Check sheet for the modelled part. Datum: model origin and axes. Units: mm. Face numbers are marked on the shaded views. A direction names the side the tool comes from. Round coordinates to 2 decimals unless told otherwise and drop trailing zeros. Order: outer loops, then holes, each group sorted by start corner. A loop starts at its lowest first (then second) coordinate and runs counter-clockwise, first axis right, second up.
(1) Sectioned sample at C-C, the plane x = 4.5. Enter the section's corners in (y, z).
(2) Thickness scan on probe 1 along Y at (x, z) = (19.5, 10); probe 2 along X at (y, z) = (-5, 19); probe 3 along Y at (x, z) = (-28.5, 9). Record the ranges inside material, lowest first.
(3) Sectioned sample at A-A, the plane y = 4. Enter the section's corners in (x, z), and give its area (3 significant figures).
(4) Sectioned sample at B-B, the plane z = 15.5. Enter the section's corners in (x, y).
(5) Depth check by flat-ended pin: pin 1 (1.5 mm diameter, centred on x = 1.5, y = 6, fed in from +Z); pin 2 (1 mm diameter, centred on x = 0.5, y = 0, fed in from -Z); pin 3 (10 mm diameter, centred on x = 8.5, y = -2.5, fed in from +Z). Enter the tip coordinate at first touch or a pass-through.
(6) Mould release check, pull along X, two halves, no side actions. Record for the marked faces 1, 2 and 3: released by +X, released by -X, zero draft, split by the parting line, or undercut.
(7) Tool access check on the marked faces 4 and 5. Record the directions out of +Z, -Z, +X, -X, +Y, -Y that give a thin tool (end or side, any length) a straight path to the whole face; none if there is none.
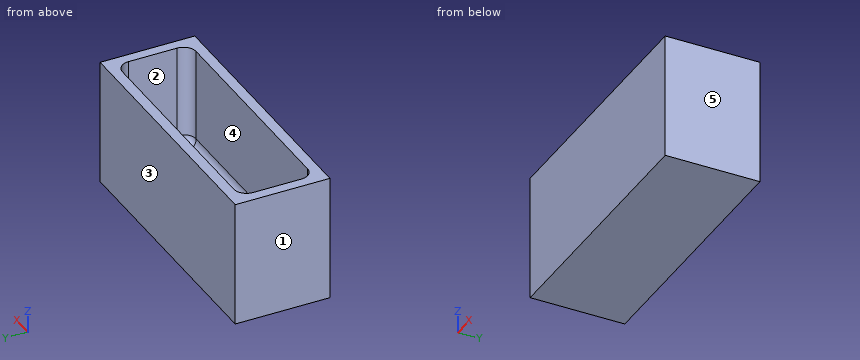
```python
from build123d import *

# Parameters (mm, degrees)
F0_W     = 79.375
F0_H     = 28.575
F1_DEPTH = 6.35
F2_W     = 79.375
F2_H     = 28.575
F2_W_2   = 73.025
F2_H_2   = 22.225
F3_DEPTH = 31.75
F4_R     = 3.81


with BuildPart() as f1:
    # F0 (on Top) → F1 (new body)
    with BuildSketch(Plane.XY):
        Rectangle(F0_W, F0_H)
    extrude(amount=F1_DEPTH)

    # F2 (on face) → F3 (join)
    with BuildSketch(Plane.XY.offset(6.35)):
        Rectangle(F2_W, F2_H)
        Rectangle(F2_W_2, F2_H_2, mode=Mode.SUBTRACT)
    extrude(amount=F3_DEPTH)

    # F4
    f4_edges = [f1.edges().sort_by_distance(p)[0] for p in [
        (0, -11.1125, 6.35),
        (-36.5125, 0, 6.35),
        (0, 11.1125, 6.35),
        (36.5125, 0, 6.35),
        (36.5125, 11.1125, 22.225),
        (36.5125, -11.1125, 22.225),
        (-36.5125, -11.1125, 22.225),
        (-36.5125, 11.1125, 22.225),
    ]]
    fillet(f4_edges, radius=F4_R)


solid = f1.part
```
Derived:
1. outline: (-14.29, 0) - (14.29, 0) - (14.29, 38.1) - (11.11, 38.1) - (11.11, 10.16) arc R3.81 cw to (7.3, 6.35) - (-7.3, 6.35) arc R3.81 cw to (-11.11, 10.16) - (-11.11, 38.1) - (-14.29, 38.1) - close
2. probe 1: y = -14.29 to -11.11, 11.11 to 14.29
2. probe 2: x = -39.69 to -36.51, 36.51 to 39.69
2. probe 3: y = -14.29 to -10.93, 10.93 to 14.29
3. outline: (-39.69, 0) - (39.69, 0) - (39.69, 38.1) - (36.51, 38.1) - (36.51, 10.16) arc R3.81 cw to (32.7, 6.35) - (-32.7, 6.35) arc R3.81 cw to (-36.51, 10.16) - (-36.51, 38.1) - (-39.69, 38.1) - close
3. area: 712 mm2
4. outline: (-39.69, -14.29) - (39.69, -14.29) - (39.69, 14.29) - (-39.69, 14.29) - close; hole (-36.51, -7.3) arc R3.81 ccw to (-32.7, -11.11) - (32.7, -11.11) arc R3.81 ccw to (36.51, -7.3) - (36.51, 7.3) arc R3.81 ccw to (32.7, 11.11) - (-32.7, 11.11) arc R3.81 ccw to (-36.51, 7.3) - close
5. pin 1: stops at z = 6.35
5. pin 2: stops at z = 0
5. pin 3: stops at z = 6.36
6. face 1: released by -X
6. face 2: undercut
6. face 3: zero draft
7. face 4: +Z
7. face 5: +Z, -Z, +X, +Y, -Y
